Design review of the part built by this model. Coordinates are the model's own, in mm. A direction names the side the tool comes from. Give positions to 0.01 mm unless a question says otherwise; leave off trailing zeros. Loops run counter-clockwise (first coordinate to the right, second up) from the corner with the lowest first, then second, coordinate; pieces in that order, holes last. Notation, with made-up numbers: (43, 51) -> (77, 51) arc R27 ccw to (77, 71) -> close; hole circle Ø5 at (-12.5, 76). An arc over 180 degrees is marked (long way). Answer in a Markdown table with one row per item. Add a question column.
(1) For pin 1 (2 mm diameter, centred on x = 0.5, y = 10, fed in from -Z), flat-tipped, find the tip position at first contact; note if it passes through.
(2) For line 1 (Y direction, x = -0.3, z = -1.4); line 2 (Z direction, x = -1.6, y = -14); line 3 (Z direction, x = -0.25, y = -4), list the stretches that pass through material, from the lowest coordinate up.
(3) Consider section A-A on z = 0. Write out the cut boundary in (x, y).
(4) For faces 1 (the flat face through (0, 31, 0)), 2 (the flat face through (-1, -25, -1)), 3 (the flat face through (-1, 25, -1)), list the 3-axis set-ups (+Z, -Z, +X, -X, +Y, -Y) from which the entire face can be reached by the end or side of a thin tool; tool diameter is ignored.
(5) Consider section C-C on x = 0.7. Write out the cut boundary in (y, z).
(6) Consider section B-B on y = 4. Write out the cut boundary in (x, z).
from build123d import *

# Parameters (mm, degrees)
EXTRUDE_1_DEPTH = 25
SKETCH_2_R      = 1.25
EXTRUDE_2_DEPTH = 31


with BuildPart() as part:
    # 草图1 → 凸台-拉伸1 (new body, symmetric)
    with BuildSketch(Plane(origin=(0, 0, 0), x_dir=(1, 0, 0), z_dir=(0, 1, 0))):
        Polygon((2.25, -1.299038106), (2.25, 1.299038106), (0, 2.598076211), (-2.25, 1.299038106), (-2.25, -1.299038106), (0, -2.598076211), align=None)
    extrude(amount=EXTRUDE_1_DEPTH, both=True)

    # 草图2 → 凸台-拉伸2 (add, symmetric)
    with BuildSketch(Plane(origin=(0, 0, 0), x_dir=(1, 0, 0), z_dir=(0, 1, 0))):
        Circle(SKETCH_2_R)
    extrude(amount=EXTRUDE_2_DEPTH, both=True)


solid = part.part
Values follow:
| question | item | result |
|---|---|---|
| 1 | pin 1 | z = -2.6 |
| 2 | line 1 | -25 to 25 |
| 2 | line 2 | -1.67 to 1.67 |
| 2 | line 3 | -2.45 to 2.45 |
| 3 | outline | (-2.25, -25) -> (-1.25, -25) -> (-1.25, -31) -> (1.25, -31) -> (1.25, -25) -> (2.25, -25) -> (2.25, 25) -> (1.25, 25) -> (1.25, 31) -> (-1.25, 31) -> (-1.25, 25) -> (-2.25, 25) -> close |
| 4 | face 1 | +Z, -Z, +X, -X, +Y |
| 4 | face 2 | -Y |
| 4 | face 3 | +Y |
| 5 | outline | (-31, -1.04) -> (-25, -1.04) -> (-25, -2.19) -> (25, -2.19) -> (25, -1.04) -> (31, -1.04) -> (31, 1.04) -> (25, 1.04) -> (25, 2.19) -> (-25, 2.19) -> (-25, 1.04) -> (-31, 1.04) -> close |
| 6 | outline | (-2.25, -1.3) -> (0, -2.6) -> (2.25, -1.3) -> (2.25, 1.3) -> (0, 2.6) -> (-2.25, 1.3) -> close |
